Part model, mm, in its own coordinate system. A direction names the side the tool comes from. Coordinates: 2 decimals unless noted, no trailing zeros. Loops run counter-clockwise (first coordinate to the right, second up) from the corner with the lowest first, then second, coordinate; pieces in that order, holes last. Notation, with made-up numbers: (40, 29) - (66, 29) arc R27 cw to (66, 57) - close; hole circle Ø1 at (81.5, 85.25). An arc over 180 degrees is marked (long way). Use a Markdown table: item, result. Add a question column.
1) Band-saw the part on C-C (z = 82.5). Give the cut face in (x, y), plus the area to 3 significant figures.
2) Band-saw the part on D-D (x = -13). Give the cut face in (y, z), plus the area to 3 significant figures.
3) Drop flat-ended pins along their axis: P1, Ø5, axis at y = 4.5, z = 44, coming from the -X side; P2, Ø5.5, axis at y = -13, z = 59, coming from the +X side; P3, Ø6, axis at x = 4, z = 17.5, coming from the -Y side. Give the stop position or say it passes through.
4) Tool access for faces 1 (the face through (3, -10, 100)), 2 (the face through (0, -12, 1)), 3 (the face through (0, -12.4, 18.5)): list every direction of +Z, -Z, +X, -X, +Y, -Y with a clear straight run to the whole face (end or side of a thin tool).
5) Band-saw the part on A-A (y = 0). Give the cut face in (x, z).
6) Band-saw the part on B-B (x = 2.5). Give the cut face in (y, z), plus the area to 3 significant figures.
7) Pull direction X, two halves, no side cores. Call faces 4 (the face through (-14.985, 0.66, 49.3)), 5 (the face through (10, -3, 0)), 6 (the face through (0, -12.4, 96.5)): +X half, -X half, draft (parallel to the pull), parting line (faces both ways), or undercut.
8) Probe probe 1 along Y at (x, z) = (0, 21); probe 2 along Z at (x, y) = (1, -12.5); probe 3 along X at (y, z) = (-8, 58). List the from-to ranges inside material, lowest first. Write a range as [from, to].
from build123d import *

# Parameters (mm, degrees)
SKETCH1_R           = 15
SKETCH1_R_2         = 10
BOSS_EXTRUDE1_DEPTH = 100
CUT_EXTRUDE1_DEPTH  = 1
CUT_EXTRUDE2_DEPTH  = 103.225241501


with BuildPart() as part:
    # Sketch1 → Boss-Extrude1 (new body)
    with BuildSketch(Plane(origin=(0, 0, 0), x_dir=(0, 1, 0), z_dir=(0, 0, 1))):
        with Locations(Location((0, 0, 0), (0, 0, 270))):
            Circle(SKETCH1_R)
        with Locations(Location((0, 0, 0), (0, 0, 270))):
            Circle(SKETCH1_R_2, mode=Mode.SUBTRACT)
    extrude(amount=BOSS_EXTRUDE1_DEPTH)

    # Sketch2 → Cut-Extrude1 (cut)
    with BuildSketch(Plane(origin=(0, 0, 0), x_dir=(-1, 0, 0), z_dir=(0, 0, -1))):
        Polygon((0, -13.732646586), (-1.577694242, -11), (1.577694242, -11), align=None)
    extrude(amount=-CUT_EXTRUDE1_DEPTH, mode=Mode.SUBTRACT)

    # Sketch4 → Cut-Extrude2 (cut, through all)
    with BuildSketch(Plane(origin=(0, 0, 0), x_dir=(-1, 0, 0), z_dir=(0, 1, 0))):
        with BuildLine():
            Line((-1.5, 20), (-1.5, 95))
            ThreePointArc((-1.5, 95), (0, 96.5), (1.5, 95))
            Line((1.5, 95), (1.5, 20))
            ThreePointArc((1.5, 20), (0, 18.5), (-1.5, 20))
        make_face()
    extrude(amount=-CUT_EXTRUDE2_DEPTH, mode=Mode.SUBTRACT)


solid = part.part
Answer block:
| question | item | result |
|---|---|---|
| 1 | outline | (-1.5, -14.92) - (-1.5, -9.89) arc R10 cw (long way) to (1.5, -9.89) - (1.5, -14.92) arc R15 ccw (long way) to start |
| 1 | area | 378 mm2 |
| 2 | outline | (-7.48, 0) - (7.48, 0) - (7.48, 100) - (-7.48, 100) - close |
| 2 | area | 1,500 mm2 |
| 3 | P1 | x = -14.87 |
| 3 | P2 | x = 10.95 |
| 3 | P3 | y = -14.97 |
| 4 | face 1 | +Z, +X, -X, +Y, -Y |
| 4 | face 2 | -Z |
| 4 | face 3 | -Y |
| 5 | outline | (-15, 0) - (-10, 0) - (-10, 100) - (-15, 100) - close; (10, 0) - (15, 0) - (15, 100) - (10, 100) - close |
| 6 | outline | (-14.79, 0) - (-9.68, 0) - (-9.68, 100) - (-14.79, 100) - close; (9.68, 0) - (14.79, 0) - (14.79, 100) - (9.68, 100) - close |
| 6 | area | 1,020 mm2 |
| 7 | face 4 | parting line |
| 7 | face 5 | draft |
| 7 | face 6 | undercut |
| 8 | probe 1 | [10, 15] |
| 8 | probe 2 | [0, 18.88], [96.12, 100] |
| 8 | probe 3 | [-12.69, -6], [6, 12.69] |
